Can you work these out from the model? Positions are in its coordinate system, mm. Coordinates: 2 decimals unless noted, no trailing zeros. Order: outer loops, then holes, each group sorted by start corner. A loop starts at its lowest first (then second) coordinate and runs counter-clockwise, first axis right, second up. Notation, with made-up numbers: (-25, -11.5) -> (-16, -11.5) arc R22 cw to (-16, -1.5) -> close; hole circle Ø3 at (19.25, 85). An arc over 180 degrees is marked (long way). Answer in a Markdown table with one row per item.
```python
from build123d import *

# Parameters (mm, degrees)
SKETCH1_R           = 14.3129
BOSS_EXTRUDE1_DEPTH = 3.175


with BuildPart() as part:
    # Sketch1 → Boss-Extrude1 (new body)
    with BuildSketch(Plane(origin=(0, 0, 0), x_dir=(1, 0, 0), z_dir=(0, 1, 0))):
        with BuildLine():
            Line((-25.4, 0), (-25.4, -250.825))
            Line((-25.4, -250.825), (141.2875, -250.825))
            Line((141.2875, -250.825), (141.2875, 0))
            Line((141.2875, 0), (134.9375, 0))
            Line((134.9375, 0), (134.9375, -225.425))
            Line((134.9375, -225.425), (25.4, -225.425))
            Line((25.4, -225.425), (25.4, 0))
            ThreePointArc((25.4, 0), (0, 25.4), (-25.4, 0))
        make_face()
        Circle(SKETCH1_R, mode=Mode.SUBTRACT)
    extrude(amount=BOSS_EXTRUDE1_DEPTH)


solid = part.part
```
(1) We'd pull the mould along Z, two halves only. Please class faces 1 (the cylindrical face through (-1.86, 1.57, -14.19)), 2 (the cylindrical face through (0.559, 1.565, -25.394)), 3 (the flat face through (20, 0, 141)): +Z half, -Z half, draft (parallel to the pull), parting line (faces both ways), or undercut.
Response values:
| item | result |
|---|---|
| face 1 | undercut |
| face 2 | -Z half |
| face 3 | draft |
(2) I need wall thicknesses on line 1 (X direction, y = 1.1, z = 196); line 2 (Z direction, x = 1, y = 1.9) (3 decimals); line 3 (Z direction, x = 79, y = 0.65) (3 decimals). Which ranges of each line are inside material? Lowest first, please. Write a range as [from, to].
Response values:
| item | result |
|---|---|
| line 1 | [-25.4, 25.4], [134.94, 141.29] |
| line 2 | [-25.38, -14.278], [14.278, 250.825] |
| line 3 | [225.425, 250.825] |
(3) Suppose I cut it at A-A (z = 23.5). Please give me the cut outline in (x, y) (1 decimal), and give its area (3 significant figures).
Response values:
| item | result |
|---|---|
| outline | (-25.4, 0) -> (25.4, 0) -> (25.4, 3.2) -> (-25.4, 3.2) -> close; (134.9, 0) -> (141.3, 0) -> (141.3, 3.2) -> (134.9, 3.2) -> close |
| area | 181 mm2 |
(4) Suppose I cut it at D-D (x = 28.5). Please give me the cut outline in (y, z) (3 decimals), and give its area (3 significant figures).
Response values:
| item | result |
|---|---|
| outline | (0, 225.425) -> (3.175, 225.425) -> (3.175, 250.825) -> (0, 250.825) -> close |
| area | 80.6 mm2 |
(5) Suppose I cut it at C-C (x = 0). Please give me the cut outline in (y, z) (3 decimals), and give its area (3 significant figures).
Response values:
| item | result |
|---|---|
| outline | (0, -25.4) -> (3.175, -25.4) -> (3.175, -14.313) -> (0, -14.313) -> close; (0, 14.313) -> (3.175, 14.313) -> (3.175, 250.825) -> (0, 250.825) -> close |
| area | 786 mm2 |
(6) Will these pins go through, and if not, where does the flat tip stop? pin 1 Ø1 at (x, y) = (90, 1) entering from -Z (3 decimals); pin 2 Ø1.6 at (x, y) = (136.5, 2) entering from -Z.
Response values:
| item | result |
|---|---|
| pin 1 | z = 225.425 |
| pin 2 | z = 0 |
(7) Suppose I cut it at B-B (y = 0.7). Please give me the cut outline in (x, z) (1 decimal).
Response values:
| item | result |
|---|---|
| outline | (-25.4, 0) arc R25.4 ccw to (25.4, 0) -> (25.4, 225.4) -> (134.9, 225.4) -> (134.9, 0) -> (141.3, 0) -> (141.3, 250.8) -> (-25.4, 250.8) -> close; hole circle Ø28.6 at (0, 0) |
